Geometry: final body of the model. Coordinates: model frame, mm. Face numbers are marked on the shaded views. Give positions to 0.01 mm unless a question says otherwise; leave off trailing zeros. Loops run counter-clockwise (first coordinate to the right, second up) from the corner with the lowest first, then second, coordinate; pieces in that order, holes last. Notation, with made-up numbers: (-12.5, 89.25) - (32.5, 89.25) arc R29 cw to (32.5, 109.25) - close; hole circle Ø4 at (39.5, 52.5). An arc over 180 degrees is marked (long way). Answer in a Markdown table with one row per item.
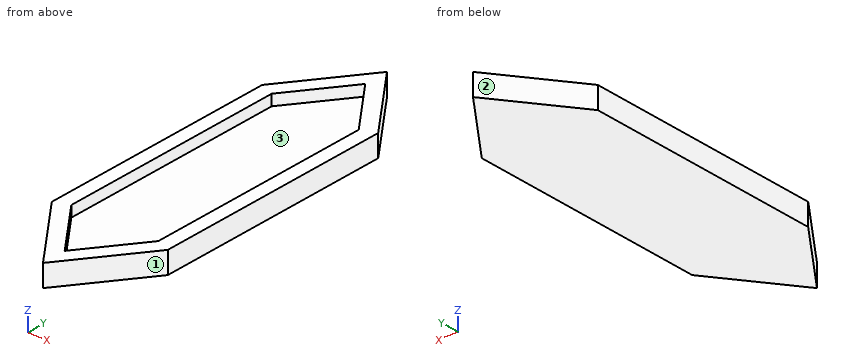
from build123d import *

# Parameters (mm, degrees)
F1_DEPTH = 9.525
F2_DEPTH = 4.7625


# Not quite as in the source:
# - a feature names something its author has since deleted; it is built from what else it names


with BuildPart() as f1:
    # F0 (on Top) → F1 (new body)
    with BuildSketch(Plane.XY):
        Polygon((0, 87.2066666667), (-25.4, 53.34), (-25.4, -53.34), (0, -87.2066666667), (25.4, -53.34), (25.4, 53.34), align=None)
        Polygon((-19.05, -50.8), (-19.05, 50.8), (0, 76.2), (19.05, 50.8), (19.05, -50.8), (0, -76.2), align=None, mode=Mode.SUBTRACT)
    extrude(amount=F1_DEPTH)

    # F0 (on Top) → F2 (join)
    with BuildSketch(Plane.XY):
        Polygon((0, 76.2), (-19.05, 50.8), (-19.05, -50.8), (0, -76.2), (19.05, -50.8), (19.05, 50.8), align=None)
    extrude(amount=F2_DEPTH)


solid = f1.part
Q1. Material intervals for line 1 along X through (y, z) = (-7, 8.5); line 2 along Z through (x, y) = (4.5, -2); line 3 along Y through (x, z) = (13, 8.75), sorted ascending.
Check values:
| item | result |
|---|---|
| line 1 | -25.4 to -19.05, 19.05 to 25.4 |
| line 2 | 0 to 4.76 |
| line 3 | -69.87 to -58.87, 58.87 to 69.87 |
Q2. Cut plane C-C (x = 10). Output: boundary loops of the cut face in (y, z) (1 decimal), and give its area (3 significant figures).
Check values:
| item | result |
|---|---|
| outline | (-73.9, 0) - (73.9, 0) - (73.9, 9.5) - (62.9, 9.5) - (62.9, 4.8) - (-62.9, 4.8) - (-62.9, 9.5) - (-73.9, 9.5) - close |
| area | 808 mm² |
Q3. Cut plane A-A (z = 7). Output: boundary loops of the cut face in (x, y), and give its area (3 significant figures).
Check values:
| item | result |
|---|---|
| outline | (-25.4, -53.34) - (0, -87.21) - (25.4, -53.34) - (25.4, 53.34) - (0, 87.21) - (-25.4, 53.34) - close; hole (-19.05, -50.8) - (0, -76.2) - (19.05, -50.8) - (19.05, 50.8) - (0, 76.2) - (-19.05, 50.8) - close |
| area | 2,300 mm² |
Q4. Draft query along X for the marked faces 1, 2 and 3. Return one class per face: pulls with the +X half, pulls with the -X half, needs draft (parallel to the pull), parting line crosses it, or undercut.
Check values:
| item | result |
|---|---|
| face 1 | pulls with the +X half |
| face 2 | pulls with the -X half |
| face 3 | undercut |
Q5. First-contact query: pin 1 (3 mm diameter, centred on x = -5, y = 26, fed in from +Z). Flat tip, straight axial feed; report the tip coordinate or a pass-through.
Check values:
| item | result |
|---|---|
| pin 1 | z = 4.76 |
